Could you check a few things on this model? Use its own coordinates, in mm. A direction names the side the tool comes from. Coordinates: 2 decimals unless noted, no trailing zeros. Order: outer loops, then holes, each group sorted by start corner. A loop starts at its lowest first (then second) coordinate and runs counter-clockwise, first axis right, second up. Notation, with made-up numbers: (-35.5, 30.5) -> (20.5, 30.5) arc R10 cw to (20.5, 44.5) -> close; hole circle Ø1 at (78.5, 78.5). An arc over 180 degrees is marked (long way). Use a Markdown table: item, result. Add a question column.
1) Which directions (+Z, -Z, +X, -X, +Y, -Y) give clear straight access to the entire face, cutting with the end or side of a thin tool? Please do faces 1 (the cylindrical face through (19.84, -18.48, 7.89)), 2 (the flat face through (15.25, 10, 8)), 3 (the cylindrical face through (-14.949, 19.715, 8.112)).
2) If we section it at D-D (x = 4.5): Write out the boundary of the cut face in (y, z).
3) Thinking about a two-plate mould opening in Y: for faces 4 (the cylindrical face through (-16.75, -18.57, 7.89)), 5 (the flat face through (1, 22, 16)), 6 (the cylindrical face through (12.051, -0.285, 8.112)), which applies, +Y half, -Y half, draft (parallel to the pull), parting line (faces both ways), or undercut?
4) If we section it at C-C (y = 4.5): Write out the boundary of the cut face in (x, z), plus the area to 3 significant figures.
5) Will this pin go through, and if not, where does the flat tip stop? pin 1 Ø3 at (x, z) = (-9, 8) entering from -Y.
6) If we section it at B-B (z = 1.75): Write out the boundary of the cut face in (x, y), plus the area to 3 significant figures.
7) If we section it at A-A (y = -11): Write out the boundary of the cut face in (x, z), plus the area to 3 significant figures.
8) If I drill on L1, parallel to X at y = -7, z = 11.75; L2, parallel to X at y = 1, z = 1; L3, parallel to Y at x = 9.5, z = 5, over which ranges is the centre line in solid material (lowest first)? Write a range as [from, to].
```python
from build123d import *

# Parameters (mm, degrees)
BOSS_EXTRUDE1_DEPTH = 16
FILLET1_R           = 5
FILLET2_R           = 1


with BuildPart() as part:
    # Sketch1 → Boss-Extrude1 (new body)
    with BuildSketch(Plane.XY):
        Polygon((15.25, 0), (11.75, 0), (11.75, -20), (21.25, -20), (21.25, 26), (-21.25, 26), (-21.25, -20), (-15.25, -20), (-15.25, 20), (15.25, 20), align=None)
    extrude(amount=BOSS_EXTRUDE1_DEPTH)

    # Fillet1
    # the kernel refuses this fillet: 5 mm, written as the material it takes off along each edge
    with BuildSketch(Plane(origin=(-15.25, -20, -12.5), x_dir=(-1, 0, 0), z_dir=(0, 0, 1)), Plane(origin=(-21.25, 26, -12.5), x_dir=(1, 0, 0), z_dir=(0, 0, 1)), Plane(origin=(21.25, 26, -12.5), x_dir=(0, -1, 0), z_dir=(0, 0, 1)), Plane(origin=(21.25, -20, -12.5), x_dir=(-1, 0, 0), z_dir=(0, 0, 1)), Plane(origin=(11.75, -20, -12.5), x_dir=(0, 1, 0), z_dir=(0, 0, 1))) as fillet1_piece_1:
        with BuildLine():
            CenterArc((FILLET1_R, -FILLET1_R), FILLET1_R, 90, 90)
            Line((0, -FILLET1_R), (0, 0))
            Line((0, 0), (FILLET1_R, 0))
        make_face()
    extrude(amount=41, mode=Mode.SUBTRACT)

    # Fillet2
    fillet2_edges = [part.edges().sort_by_distance(p)[0] for p in [
        (11.75, 0, 8),
        (15.25, 0, 8),
        (15.25, 20, 8),
        (-15.25, 20, 8),
    ]]
    fillet(fillet2_edges, radius=FILLET2_R)


solid = part.part
```
Answer sheet:
| question | item | result |
|---|---|---|
| 1 | face 1 | +Z, -Z, +X, -Y |
| 1 | face 2 | +Z, -Z |
| 1 | face 3 | +Z, -Z, -Y |
| 2 | outline | (20, 0) -> (26, 0) -> (26, 16) -> (20, 16) -> close |
| 3 | face 4 | -Y half |
| 3 | face 5 | draft |
| 3 | face 6 | undercut |
| 4 | outline | (-21.25, 0) -> (-15.25, 0) -> (-15.25, 16) -> (-21.25, 16) -> close; (15.25, 0) -> (21.25, 0) -> (21.25, 16) -> (15.25, 16) -> close |
| 4 | area | 192 mm2 |
| 5 | pin 1 | y = 20 |
| 6 | outline | (-21.25, -20) -> (-20.25, -20) arc R5 ccw to (-15.25, -15) -> (-15.25, 19) arc R1 cw to (-14.25, 20) -> (14.25, 20) arc R1 cw to (15.25, 19) -> (15.25, 1) arc R1 cw to (14.25, 0) -> (12.75, 0) arc R1 ccw to (11.75, -1) -> (11.75, -15) arc R5 ccw to (16.5, -19.99) arc R5 ccw to (21.25, -15) -> (21.25, 21) arc R5 ccw to (16.25, 26) -> (-16.25, 26) arc R5 ccw to (-21.25, 21) -> close |
| 6 | area | 779 mm2 |
| 7 | outline | (-21.25, 0) -> (-15.25, 0) -> (-15.25, 16) -> (-21.25, 16) -> close; (11.75, 0) -> (21.25, 0) -> (21.25, 16) -> (11.75, 16) -> close |
| 7 | area | 248 mm2 |
| 8 | L1 | [-21.25, -15.25], [11.75, 21.25] |
| 8 | L2 | [-21.25, -15.25], [15.25, 21.25] |
| 8 | L3 | [20, 26] |
